Geometry: final body of the model. Coordinates: model frame, mm. A direction names the side the tool comes from. Coordinates: 2 decimals unless noted, no trailing zeros. Write each loop counter-clockwise with the first axis right and the second up, starting at its lowest first coordinate (ties: lowest second). Pieces come first, ordered by that corner, then holes. Notation, with made-up numbers: (-12.5, 46.25) - (15.5, 46.25) arc R6 cw to (15.5, 56.25) - close; hole circle Ø7 at (61.5, 85.25). An arc over 180 degrees is marked (long way). Answer as a JSON object with one key per item and string values. Group by question number.
Item 1: First-contact query: pin 1 Ø6 at (y, z) = (11.5, -59.5) entering from -X; pin 2 Ø12 at (x, y) = (27, 44.5) entering from +Z; pin 3 Ø2 at (y, z) = (-27, 20.5) entering from -X. Flat tips, straight axial feed; report the tip coordinate or a pass-through.
Item 2: Section B-B on y = 110. Return loops of the section in (x, z), and give its area (3 significant figures).
Item 3: Line query: line 1 along Y through (x, z) = (-25, 38); line 2 along Y through (x, z) = (36, -15); line 3 along Y through (x, z) = (43.5, -80). Output: solid intervals per line, ascending. Write a range as from..to.
Item 4: Set-up query: faces 1 (the flat face through (-8, 0, 80)), 2 (the flat face through (-1, -50, 1)). Return all of +Z, -Z, +X, -X, +Y, -Y with unobstructed straight access to the full face (end or side cutting, diameter ignored); none if empty.
Item 5: Section A-A on y = -33. Return loops of the section in (x, z).
```python
from build123d import *

# Parameters (mm, degrees)
ESQUISSE2_R      = 100
EXTRUSION1_DEPTH = 50
CHANFREIN1_SIZE  = 2.5


with BuildPart() as part:
    # Esquisse1 → Révolution2 (revolve)
    with BuildSketch(Plane.XY):
        with BuildLine():
            Line((0, 160), (-30, 160))
            ThreePointArc((-30, 160), (-50, 140), (-30, 120))
            ThreePointArc((-30, 120), (-5, 95), (-30, 70))
            ThreePointArc((-30, 70), (-65.355339059, 55.355339059), (-80, 20))
            Line((-80, 20), (-80, 0))
            Line((-80, 0), (0, 0))
            Line((0, 0), (0, 160))
        make_face()
    revolve(axis=Axis((0, 160, 0), (0, -1, 0)))

    # Esquisse2 → Extrusion1 (add)
    with BuildSketch(Plane.XZ):
        Circle(ESQUISSE2_R)
    extrude(amount=EXTRUSION1_DEPTH)

    # Chanfrein1
    chanfrein1_edges = [part.edges().sort_by_distance(p)[0] for p in [
        (-100, 0, 0),
        (-100, -50, 0),
    ]]
    chamfer(chanfrein1_edges, length=CHANFREIN1_SIZE)


solid = part.part
```
Checks:
{
 "1": {"pin 1": "x = -56.64", "pin 2": "z = 72.26", "pin 3": "x = -98.08"},
 "2": {"outline": "circle Ø20 at (0, 0)", "area": "314 mm^2"},
 "3": {"line 1": "-50..67.54, 127.34..152.66", "line 2": "-50..69.18, 122.14..157.86", "line 3": "-50..0"},
 "4": {"face 1": "+Y", "face 2": "+Z, -Z, +X, -X, -Y"},
 "5": {"outline": "circle Ø200 at (0, 0)"}
}
